Can you work these out from the model? Positions are in its coordinate system, mm. A direction names the side the tool comes from. Round coordinates to 2 decimals unless told otherwise and drop trailing zeros. Loops run counter-clockwise (first coordinate to the right, second up) from the corner with the lowest first, then second, coordinate; pieces in that order, holes last.
from build123d import *

# Parameters (mm, degrees)
PAD_DEPTH    = 17
POCKET_DEPTH = 15
FILLET_R     = 2


with BuildPart() as part:
    # Sketch → Pad (new body)
    with BuildSketch(Plane.XY):
        with BuildLine():
            Line((7, 0), (42, 0))
            ThreePointArc((42, 0), (46.976998, 2.077654), (48.999573, 7.077287))
            Line((48.999573, 7.077287), (48.999573, 12))
            Line((30, 42), (48.999573, 12))
            Line((30, 42), (18, 42))
            ThreePointArc((18, 42), (5.270984, 36.726828), (0, 23.996906))
            Line((0, 23.996906), (0, 7.00193))
            ThreePointArc((0, 7.00193), (2.04957, 2.050935), (7, 0))
        make_face()
    extrude(amount=PAD_DEPTH)

    # Sketch001 → Pocket (cut)
    with BuildSketch(Plane.XY.offset(17)):
        with BuildLine():
            Line((6.887434, 2.001267), (42.011518, 2.001267))
            ThreePointArc((42.011518, 2.001267), (45.614855, 3.546862), (46.99536, 7.216617))
            Line((46.99536, 7.216617), (46.99536, 12))
            Line((29, 40), (46.99536, 12))
            Line((29, 40), (17.998587, 40))
            ThreePointArc((17.998587, 40), (6.674789, 35.302194), (2.00003, 23.968863))
            Line((2.00003, 23.968863), (2.00003, 6.982594))
            ThreePointArc((2.00003, 6.982594), (3.430979, 3.498273), (6.887434, 2.001267))
        make_face()
    extrude(amount=-POCKET_DEPTH, mode=Mode.SUBTRACT)

    # Fillet
    fillet_edges = [part.edges().sort_by_distance(p)[0] for p in [
        (48.999573, 12, 8.5),
        (30, 42, 8.5),
    ]]
    fillet(fillet_edges, radius=FILLET_R)


solid = part.part
(1) If we section it at C-C, the plane x = 22: List the corners of the cut face in (y, z) for me.
Worked answers:
outline: (0, 0) - (42, 0) - (42, 17) - (40, 17) - (40, 2) - (2, 2) - (2, 17) - (0, 17) - close
(2) Will these pins go through, and if not, where does the flat tip stop? P1, Ø4.5, axis at x = 31.5, z = 9.5, coming from the +Y side; P2, Ø1.5, axis at x = 31, y = 28.5, coming from the +Z side.
Worked answers:
P1: stops at y = 41.97
P2: stops at z = 2
(3) If we section it at B-B, the plane y = 10: List the corners of the cut face in (x, z) for me, then the cut area to 3 significant figures.
Worked answers:
outline: (0, 0) - (49, 0) - (49, 17) - (47, 17) - (47, 2) - (2, 2) - (2, 17) - (0, 17) - close
area: 158 mm2
(4) If we mould it in two halves opening along Y, with no side actions, what happens to faces 3 (the cylindrical face through (29.876, 41.745, 8.619)), 4 (the flat face through (24, 0, 8)), 5 (the flat face through (24, 40, 10)), 6 (the flat face through (23, 1, 17))? For each: released by +Y, released by -Y, zero draft, split by the parting line, or undercut.
Worked answers:
face 3: released by +Y
face 4: released by -Y
face 5: undercut
face 6: zero draft
(5) For faces 1 (the cylindrical face through (48.923, 11.969, 8.619)), 2 (the cylindrical face through (6.8, 35.426, 9.605)), which set-ups out of +Z, -Z, +X, -X, +Y, -Y let a thin tool reach every point of the face, with its end or its side?
Worked answers:
face 1: +Z, -Z, +X, +Y
face 2: +Z
(6) If we section it at A-A, the plane z = 11.75: List the corners of the cut face in (x, y) for me, then the cut area to 3 significant figures.
Worked answers:
outline: (0, 7) arc R7 ccw to (7, 0) - (42, 0) arc R7 ccw to (49, 7.08) - (49, 11.42) arc R2 ccw to (48.69, 12.49) - (30.59, 41.07) arc R2 ccw to (28.9, 42) - (18, 42) arc R18 ccw to (0, 24) - close; hole (2, 6.98) arc R5 ccw to (6.89, 2) - (42.01, 2) arc R5 ccw to (47, 7.22) - (47, 12) - (29, 40) - (18, 40) arc R16 ccw to (2, 23.97) - close
area: 290 mm2
(7) If I drill on line 1 (Y direction, x = 22, z = 13); line 2 (X direction, y = 7.5, z = 11.25); line 3 (Z direction, x = 35.5, y = 22), over which ranges is the centre line in solid material (lowest first)?
Worked answers:
line 1: y = 0 to 2, 40 to 42
line 2: x = 0 to 2, 47 to 49
line 3: z = 0 to 2
